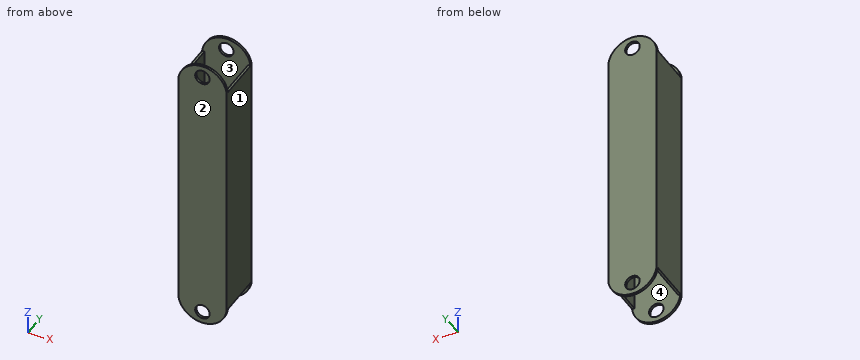
from build123d import *

# Parameters (mm, degrees)
SKETCH1_W               = 20
SKETCH1_H               = 20
SKETCH1_W_2             = 18
SKETCH1_H_2             = 18
BOSS_EXTRUDE1_DEPTH     = 50
BOSS_EXTRUDE2_START     = -1
SKETCH2_R               = 3
BOSS_EXTRUDE2_DEPTH     = 1
MIRROR2_START           = -1
MIRROR2_COPY_1_SKETCH_R = 3
MIRROR2_COPY_1_DEPTH    = 1


with BuildPart() as part:
    # Sketch1 → Boss-Extrude1 (new body, symmetric)
    with BuildSketch(Plane.XY):
        Rectangle(SKETCH1_W, SKETCH1_H)
        Rectangle(SKETCH1_W_2, SKETCH1_H_2, mode=Mode.SUBTRACT)
    extrude(amount=BOSS_EXTRUDE1_DEPTH, both=True)

    # Sketch2 → Boss-Extrude2 (add)
    with BuildSketch(Plane.XZ.offset(10).offset(BOSS_EXTRUDE2_START)):
        with BuildLine():
            Line((-10, 50), (10, 50))
            ThreePointArc((10, 50), (0, 59.049875621), (-10, 50))
        make_face()
        with Locations((0, 54)):
            Circle(SKETCH2_R, mode=Mode.SUBTRACT)
    boss_extrude2 = extrude(amount=BOSS_EXTRUDE2_DEPTH)

    # Mirror1: Boss-Extrude2 across plane
    add(boss_extrude2.mirror(Plane.XY))

    # Mirror2: Boss-Extrude2 across plane
    add(boss_extrude2.mirror(Plane.ZX))

    # Mirror2 copy 1 sketch → Mirror2 copy 1 (add)
    with BuildSketch(Plane(origin=(0, 10, 0), x_dir=(1, 0, 0), z_dir=(0, 1, 0)).offset(MIRROR2_START)):
        with BuildLine():
            Line((-10, 50), (10, 50))
            ThreePointArc((10, 50), (0, 59.049875621), (-10, 50))
        make_face()
        with Locations((0, 54)):
            Circle(MIRROR2_COPY_1_SKETCH_R, mode=Mode.SUBTRACT)
    extrude(amount=MIRROR2_COPY_1_DEPTH)


solid = part.part
Build history of the part. All positions in model axes, mm. Face numbers are marked on the shaded views. Coordinates: 2 decimals unless noted, no trailing zeros. Write each loop counter-clockwise with the first axis right and the second up, starting at its lowest first coordinate (ties: lowest second). Pieces come first, ordered by that corner, then holes. Notation, with made-up numbers: (-7.5, -31) -> (29.5, -31) arc R24 cw to (29.5, -14) -> close; hole circle Ø8 at (42.25, 4). An arc over 180 degrees is marked (long way). Use CSV: the item, a comma, the result in double quotes. Start each with the question number.
Q1. Cut at B-B, the plane x = -1.5. List the corners of the cut face in (y, z), then the cut area to 3 significant figures.
Q2. Cut at D-D, the plane z = 54. List the corners of the cut face in (x, y), then the cut area to 3 significant figures.
Q3. Drill centre lines: probe 1 along Z at (x, y) = (0, 9.75); probe 2 along X at (y, z) = (1.5, 33). Where is each one in solid material? Low to high.
Q4. Flat gauge pins, fed straight in: pin 1 Ø0.8 at (x, y) = (9.5, 1.5) entering from -Z; pin 2 Ø0.5 at (x, y) = (9.5, -3) entering from +Z; pin 3 Ø10 at (x, y) = (7, -8) entering from +Z. Where does each tip first touch, or does it go through?
Q5. Cut at C-C, the plane z = 11. List the corners of the cut face in (x, y).
Q6. Pull direction X, two halves, no side cores. Call the marked faces 1, 2, 3 and 4: released by +X, released by -X, zero draft, split by the parting line, or undercut.
Q7. Cut at A-A, the plane y = 5.25. List the corners of the cut face in (x, z), then the cut area to 3 significant figures.
Checked values:
1,outline,"(-10, -58.94) -> (-9, -58.94) -> (-9, -56.6) -> (-10, -56.6) -> close; (-10, -51.4) -> (-9, -51.4) -> (-9, 51.4) -> (-10, 51.4) -> close; (-10, 56.6) -> (-9, 56.6) -> (-9, 58.94) -> (-10, 58.94) -> close; (9, -58.94) -> (10, -58.94) -> (10, -56.6) -> (9, -56.6) -> close; (9, -51.4) -> (10, -51.4) -> (10, 51.4) -> (9, 51.4) -> close; (9, 56.6) -> (10, 56.6) -> (10, 58.94) -> (9, 58.94) -> close"
1,area,"215 mm²"
2,outline,"(-8.72, -10) -> (-3, -10) -> (-3, -9) -> (-8.72, -9) -> close; (-8.72, 9) -> (-3, 9) -> (-3, 10) -> (-8.72, 10) -> close; (3, -10) -> (8.72, -10) -> (8.72, -9) -> (3, -9) -> close; (3, 9) -> (8.72, 9) -> (8.72, 10) -> (3, 10) -> close"
2,area,"22.9 mm²"
3,probe 1,"z = -59.05 to -57, -51 to 51, 57 to 59.05"
3,probe 2,"x = -10 to -9, 9 to 10"
4,pin 1,"stops at z = -50"
4,pin 2,"stops at z = 50"
4,pin 3,"stops at z = 58.83"
5,outline,"(-10, -10) -> (10, -10) -> (10, 10) -> (-10, 10) -> close; hole (-9, -9) -> (9, -9) -> (9, 9) -> (-9, 9) -> close"
6,face 1,"released by +X"
6,face 2,"zero draft"
6,face 3,"undercut"
6,face 4,"undercut"
7,outline,"(-10, -50) -> (-9, -50) -> (-9, 50) -> (-10, 50) -> close; (9, -50) -> (10, -50) -> (10, 50) -> (9, 50) -> close"
7,area,"200 mm²"
